Job drawing, mm, ordinate dimensions from the low corner. One solid piece. A direction names the side the tool comes from. Round coordinates to 2 decimals unless told otherwise and drop trailing zeros. Loops run counter-clockwise (first coordinate to the right, second up) from the corner with the lowest first, then second, coordinate; pieces in that order, holes last. Notation, with made-up numbers: (26, 73.5) - (75, 73.5) arc R28 ccw to (75, 100.5) - close; hole circle Ø1 at (61.25, 70). An arc over 180 degrees is marked (long way). One line per question, with ' | ' between items. Start each with the question number.
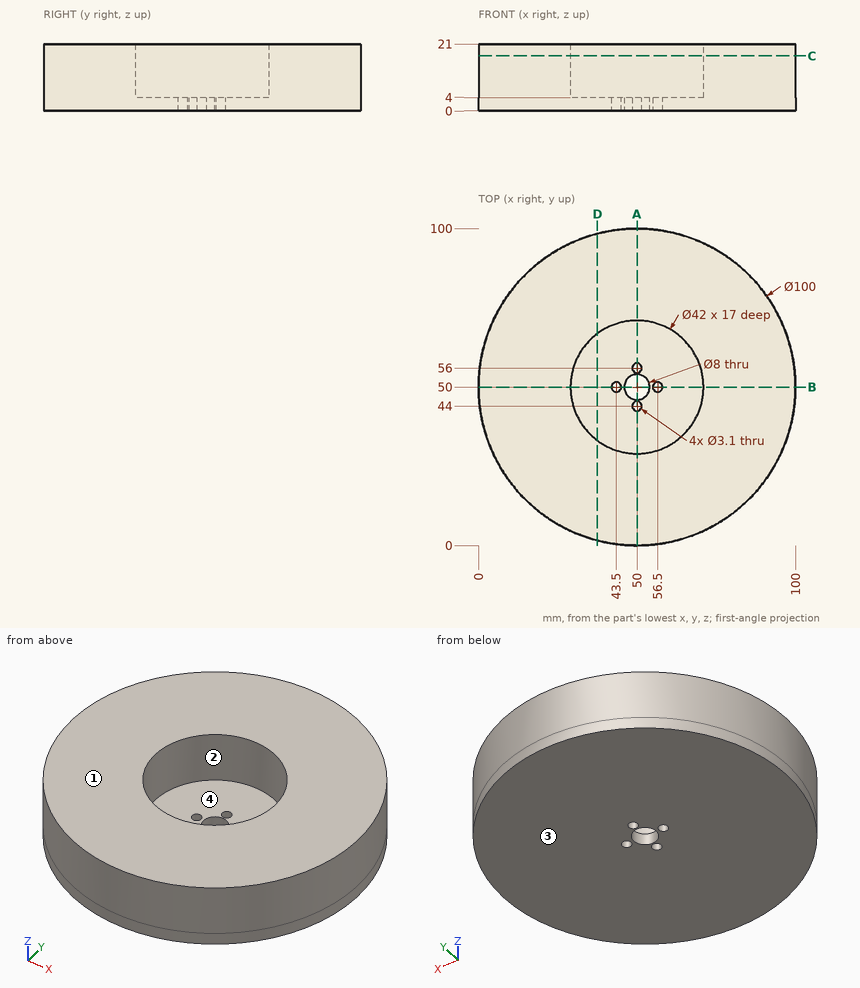
1) Tool access for the marked faces 1 and 2: list every direction of +Z, -Z, +X, -X, +Y, -Y with a clear straight run to the whole face (end or side of a thin tool).
2) Two-plate mould, pull along X, no slides. Class the marked faces 3 and 4: +X half, -X half, draft (parallel to the pull), parting line (faces both ways), or undercut.
3) Drop flat-ended pins along their axis: pin 1 (2.5 mm diameter, centred on x = 56.5, y = 50, fed in from -Z); pin 2 (10.5 mm diameter, centred on x = 50, y = 50, fed in from +Z); pin 3 (8 mm diameter, centred on y = 55.5, z = 2.5, fed in from -X); pin 4 (10 mm diameter, centred on y = 12, z = 10, fed in from +X). Give the stop position or say it passes through.
4) Saw through at D-D on x = 37.5. Write the cut outline in (y, z).
5) Saw through at C-C on z = 17.25. Write the cut outline in (x, y), and give its area (3 significant figures).
6) Saw through at A-A on x = 50. Write the cut outline in (y, z).
7) Wall check: line 1 (X direction, y = 50, z = 1.2); line 2 (Y direction, x = 50, z = 2); line 3 (X direction, y = 51, z = 7.5). Give the ranges that are in metal, low to high. Write a range as [from, to].
8) Saw through at B-B on y = 50. Write the cut outline in (x, z), and give its area (3 significant figures).
Answer key:
1) face 1: +Z, +X, -X, +Y, -Y | face 2: +Z
2) face 3: draft | face 4: undercut
3) pin 1: through | pin 2: z = 4 | pin 3: x = 0.02 | pin 4: x = 87.56
4) outline: (1.59, 0) - (98.41, 0) - (98.41, 21) - (66.87, 21) - (66.87, 4) - (33.13, 4) - (33.13, 21) - (1.59, 21) - close
5) outline: circle Ø100 at (50, 50); hole circle Ø42 at (50, 50) | area: 6,470 mm²
6) outline: (0, 0) - (42.45, 0) - (42.45, 4) - (29, 4) - (29, 21) - (0, 21) - close; (45.55, 0) - (46, 0) - (46, 4) - (45.55, 4) - close; (54, 0) - (54.45, 0) - (54.45, 4) - (54, 4) - close; (57.55, 0) - (100, 0) - (100, 21) - (71, 21) - (71, 4) - (57.55, 4) - close
7) line 1: [0, 41.95], [45.05, 46], [54, 54.95], [58.05, 100] | line 2: [0, 42.45], [45.55, 46], [54, 54.45], [57.55, 100] | line 3: [0.01, 29.02], [70.98, 99.99]
8) outline: (0, 0) - (41.95, 0) - (41.95, 4) - (29, 4) - (29, 21) - (0, 21) - close; (45.05, 0) - (46, 0) - (46, 4) - (45.05, 4) - close; (54, 0) - (54.95, 0) - (54.95, 4) - (54, 4) - close; (58.05, 0) - (100, 0) - (100, 21) - (71, 21) - (71, 4) - (58.05, 4) - close | area: 1,330 mm²
